```python
from build123d import *

# Parameters (mm, degrees)
IZIM1_R                     = 35
Y_KSEKLIK_EKSTR_ZYON1_DEPTH = 25
IZIM2_R                     = 2
KES_EKSTR_ZYON1_DEPTH       = 9
RADYUS1_R                   = 10
RADYUS2_R                   = 10


with BuildPart() as part:
    # Çizim1 → Yükseklik-Ekstrüzyon1 (new body)
    with BuildSketch(Plane.XY):
        Circle(IZIM1_R)
    extrude(amount=Y_KSEKLIK_EKSTR_ZYON1_DEPTH)

    # Çizim2 → Kes-Ekstrüzyon1 (cut)
    with BuildSketch(Plane.XY.offset(25)):
        Circle(IZIM2_R)
    extrude(amount=-KES_EKSTR_ZYON1_DEPTH, mode=Mode.SUBTRACT)

    # Radyus1
    radyus1_edges = [part.edges().sort_by_distance(p)[0] for p in [
        (-35, 0, 0),
    ]]
    fillet(radyus1_edges, radius=RADYUS1_R)

    # Radyus2
    radyus2_edges = [part.edges().sort_by_distance(p)[0] for p in [
        (-35, 0, 25),
    ]]
    fillet(radyus2_edges, radius=RADYUS2_R)


solid = part.part
```
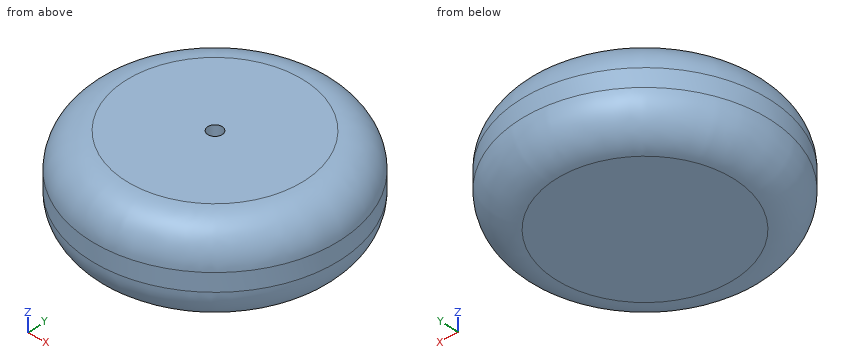
For this review, take the finished solid that the model builds, in its own axes (mm). Coordinates: 2 decimals unless noted, no trailing zeros. Loops run counter-clockwise (first coordinate to the right, second up) from the corner with the lowest first, then second, coordinate; pieces in that order, holes last. Notation, with made-up numbers: (-17, 77) - (34, 77) arc R13 ccw to (34, 92) - close; hole circle Ø7 at (68, 1.25). An arc over 180 degrees is marked (long way). Use one line per item in the form item = value. Start each with the question number.
1) Take a section at C-C (z = 11.75). State the section outline as (x, y) points.
2) For pin 1 (3 mm diameter, centred on x = 0.5, y = -0.5, fed in from +Z); pin 2 (12 mm diameter, centred on y = 11, z = 19.5, fed in from +X); pin 3 (2 mm diameter, centred on y = -17.5, z = 13.5, fed in from -X); pin 4 (1.5 mm diameter, centred on x = -17.5, y = -27, fed in from -Z), all flat-tipped, find the tip position at first contact; note any pin that passes through.
3) Take a section at D-D (z = 17.5). State the section outline as (x, y) points, plus the area to 3 significant figures.
4) To check wall thickness, follow probe 1 along Z at (x, y) = (-24, -9); probe 2 along Y at (x, z) = (-3.5, 4.25); probe 3 along Y at (x, z) = (10.5, 10.5). State the ranges of each line that lie inside material, in increasing order. Write a range as from..to.
5) Take a section at A-A (y = 0). State the section outline as (x, z) points, plus the area to 3 significant figures.
From the geometry:
q1.outline = circle Ø70 at (0, 0)
q2.pin_1 = 25
q2.pin_2 = 34.41
q2.pin_3 = -30.87
q2.pin_4 = 2.34
q3.outline = circle Ø69.36 at (0, 0); hole circle Ø4 at (0, 0)
q3.area = 3,770 mm2
q4.probe_1 = 0.02..24.98
q4.probe_2 = -33..33
q4.probe_3 = -33.39..33.39
q5.outline = (-35, 10) arc R10 ccw to (-25, 0) - (25, 0) arc R10 ccw to (35, 10) - (35, 15) arc R10 ccw to (25, 25) - (2, 25) - (2, 16) - (-2, 16) - (-2, 25) - (-25, 25) arc R10 ccw to (-35, 15) - close
q5.area = 1,630 mm2
